Drawing for the job (mm, zero at the part's lowest x, y, z). A direction names the side the tool comes from. Round coordinates to 2 decimals unless told otherwise and drop trailing zeros. Loops run counter-clockwise (first coordinate to the right, second up) from the corner with the lowest first, then second, coordinate; pieces in that order, holes last. Notation, with made-up numbers: (31, -36) - (85, -36) arc R18 cw to (85, -11) - close; hole circle Ø9 at (-23, 24.5). An arc over 180 degrees is marked (long way). Put each result on its own line as item: value.
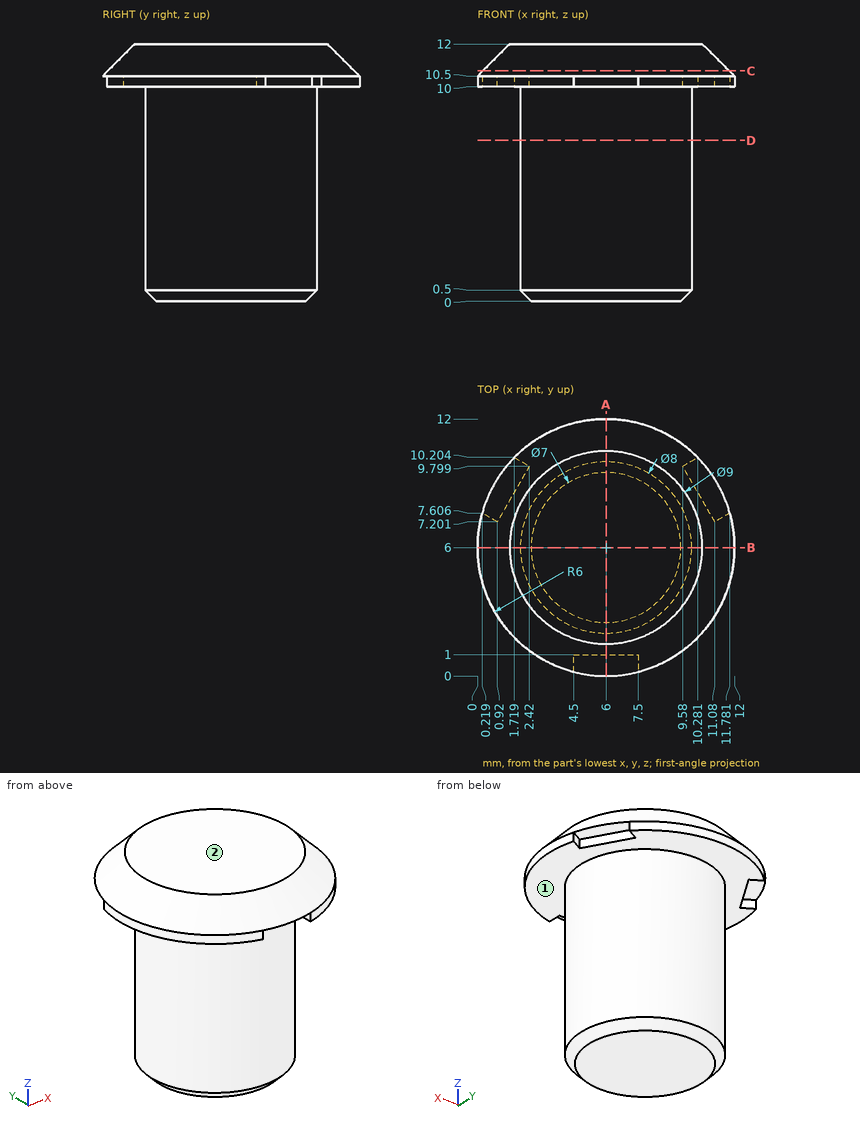
1. Probe line 1 along Z through (x, y) = (3.25, 10.75); line 2 along X through (y, z) = (9, 3) (1 decimal); line 3 along Z through (x, y) = (9.5, 2) (1 decimal). List the from-to ranges inside material, lowest first. Write a range as [from, to].
A:
line 1: z = [10, 11.01]
line 2: x = [3.4, 8.6]
line 3: z = [10, 11.2]
2. Tool access for the marked faces 1 and 2: list every direction of +Z, -Z, +X, -X, +Y, -Y with a clear straight run to the whole face (end or side of a thin tool).
A:
face 1: -Z
face 2: +Z, +X, -X, +Y, -Y
3. Band-saw the part on B-B (y = 6). List the corners of the cut face in (x, z).
A:
outline: (0, 10) - (2, 10) - (2, 0.5) - (2.5, 0) - (9.5, 0) - (10, 0.5) - (10, 10) - (12, 10) - (12, 10.5) - (10.5, 12) - (1.5, 12) - (0, 10.5) - close
4. Pin check, flat tips, straight feed: P1, Ø3, axis at x = 10, z = 3.5, coming from the +Y side; P2, Ø4, axis at y = 8, z = 5, coming from the -X side; P3, Ø2.5, axis at x = 10.5, y = 9, coming from the -Z side. Stop position of each tip, or through.
A:
P1: stops at y = 9.12
P2: stops at x = 2
P3: stops at z = 10
5. Band-saw the part on A-A (x = 6). List the corners of the cut face in (y, z).
A:
outline: (0, 10.5) - (1, 10.5) - (1, 10) - (2, 10) - (2, 0.5) - (2.5, 0) - (9.5, 0) - (10, 0.5) - (10, 10) - (12, 10) - (12, 10.5) - (10.5, 12) - (1.5, 12) - close
6. Band-saw the part on D-D (z = 7.5). List the corners of the cut face in (x, y), plus the area to 3 significant figures.
A:
outline: circle Ø8 at (6, 6)
area: 50.3 mm²
7. Band-saw the part on C-C (z = 10.75). List the corners of the cut face in (x, y).
A:
outline: circle Ø11.5 at (6, 6)
